```python
from build123d import *

# Parameters (mm, degrees)
BOX002_W            = 15
BOX002_H            = 10
BOX002_DEPTH        = 2
BOX003_W            = 3
BOX003_H            = 10
BOX003_DEPTH        = 10
BOX004_W            = 2
BOX004_H            = 10
BOX004_DEPTH        = 1
BOX001_W            = 1
BOX001_H            = 10
BOX001_DEPTH        = 10
CONE_PITCH_ANGLE    = -15
CYLINDER_R          = 2
CYLINDER_DEPTH      = 10
CYLINDER_ROLL_ANGLE = 90
BOX_W               = 10
BOX_H               = 10
BOX_DEPTH           = 1


with BuildPart() as cubo002:
    # Box002 → Box002 (new body)
    with BuildSketch(Plane(origin=(-3, 0, -2), x_dir=(1, 0, 0), z_dir=(0, 0, 1))):
        with Locations((7.5, 5)):
            Rectangle(BOX002_W, BOX002_H)
    extrude(amount=BOX002_DEPTH)


with BuildPart() as cubo003:
    # Box003 → Box003 (new body)
    with BuildSketch(Plane(origin=(-3, 0, 0), x_dir=(1, 0, 0), z_dir=(0, 0, 1))):
        with Locations((1.5, 5)):
            Rectangle(BOX003_W, BOX003_H)
    extrude(amount=BOX003_DEPTH)


with BuildPart() as cubo004:
    # Box004 → Box004 (new body)
    with BuildSketch(Plane(origin=(10, 0, 0), x_dir=(1, 0, 0), z_dir=(0, 0, 1))):
        with Locations((1, 5)):
            Rectangle(BOX004_W, BOX004_H)
    extrude(amount=BOX004_DEPTH)


with BuildPart() as cubo001:
    # Box001 → Box001 (new body)
    with BuildSketch(Plane.XY):
        with Locations((0.5, 5)):
            Rectangle(BOX001_W, BOX001_H)
    extrude(amount=BOX001_DEPTH)


with BuildPart() as cono:
    # Cone → Cone (revolve)
    with BuildSketch(Plane.XZ):
        Polygon((0, 0), (1, 0), (0.5, 5), (0, 5), align=None)
    revolve(axis=Axis((0, 0, 0), (0, 0, 1)))


with BuildPart() as cono_1:
    # Cone pitch: moved
    add(cono.part.rotate(Axis((0, 0, 0), (0, 1, 0)), CONE_PITCH_ANGLE))


with BuildPart() as cono_2:
    # Cone placement: moved
    add(cono_1.part.moved(Location((9.3, 5, 0))))


with BuildPart() as cilindro:
    # Cylinder → Cylinder (new body)
    with BuildSketch(Plane.XY):
        Circle(CYLINDER_R)
    extrude(amount=CYLINDER_DEPTH)


with BuildPart() as cilindro_1:
    # Cylinder roll: moved
    add(cilindro.part.rotate(Axis((0, 0, 0), (1, 0, 0)), CYLINDER_ROLL_ANGLE))


with BuildPart() as cilindro_2:
    # Cylinder placement: moved
    add(cilindro_1.part.moved(Location((0.5, 10, 0.5))))


with BuildPart() as cut002:
    # Box → Box (new body)
    with BuildSketch(Plane.XY):
        with Locations((5, 5)):
            Rectangle(BOX_W, BOX_H)
    extrude(amount=BOX_DEPTH)

    # Fusion: union Cubo001, Cono, Cilindro
    add(cubo001.part)
    add(cono_2.part)
    add(cilindro_2.part)

    # Cut: cut Cubo004
    add(cubo004.part, mode=Mode.SUBTRACT)

    # Cut001: cut Cubo003
    add(cubo003.part, mode=Mode.SUBTRACT)

    # Cut002: cut Cubo002
    add(cubo002.part, mode=Mode.SUBTRACT)


solid = cut002.part
```
The listing builds one solid part. Answer for the finished solid, in the listing's coordinates (mm). Round coordinates to 2 decimals unless told otherwise and drop trailing zeros. Write each loop counter-clockwise with the first axis right and the second up, starting at its lowest first coordinate (ties: lowest second). Pieces come first, ordered by that corner, then holes. Notation, with made-up numbers: (-16.5, -21.75) -> (20.5, -21.75) arc R12 cw to (20.5, -13.75) -> close; hole circle Ø6 at (53.25, 23). An arc over 180 degrees is marked (long way). Use CSV: the item, a comma, the result in double quotes. Start each with the question number.
(1) Section B-B on z = 8.75 is taken. Give the vertices of the cut face in (x, y), then the cut area to 3 significant figures.
(2) Consider L1, parallel to Z at x = 8, y = 1; L2, parallel to X at y = 5.25, z = 4.25. Determine where each line is inside the solid, lowest interval first. Write a range as from..to.
(3) The mould has two halves that part along X. Classify faces 1 (the face through (0, 5, 5)), 2 (the face through (8, 5.01, 4.83)), 3 (the face through (0.5, 5.1, 10)): released by +X, released by -X, zero draft, split by the parting line, or undercut.
(4) Each of these flat-tipped pins is pushed along its axis until it touches: pin 1 (1.5 mm diameter, centred on x = 6, y = 8, fed in from +Z); pin 2 (4 mm diameter, centred on y = 7.5, z = 8, fed in from +X). Where does it stop, or does it pass through?
(5) Section A-A on y = 8.75 is taken. Give the vertices of the cut face in (x, z), then the cut area to 3 significant figures.
(6) Section C-C on x = 7.25 is taken. Give the vertices of the cut face in (y, z), then the cut area to 3 significant figures.
A:
1,outline,"(0, 0) -> (1, 0) -> (1, 10) -> (0, 10) -> close"
1,area,"10.0 mm²"
2,L1,"z = 0..1"
2,L2,"x = 0..1, 7.66..8.7"
3,face 1,"released by -X"
3,face 2,"undercut"
3,face 3,"zero draft"
4,pin 1,"stops at z = 1"
4,pin 2,"stops at x = 1"
5,outline,"(0, 0) -> (10, 0) -> (10, 1) -> (2.44, 1) arc R2 ccw to (1, 2.44) -> (1, 10) -> (0, 10) -> close"
5,area,"20.4 mm²"
6,outline,"(0, 0) -> (10, 0) -> (10, 1) -> (0, 1) -> close"
6,area,"10.0 mm²"
